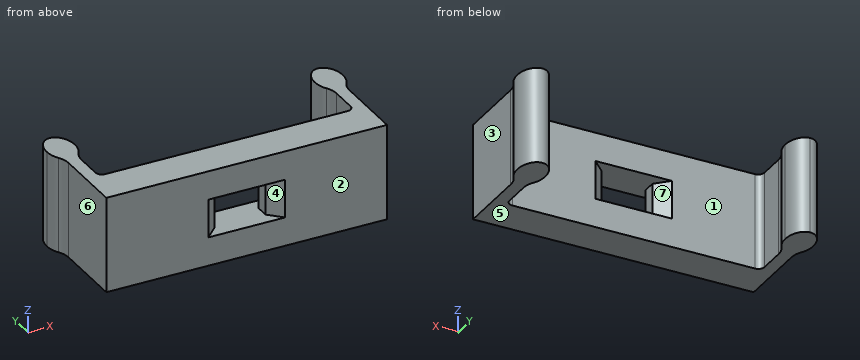
Autodesk Fusion 360 part; units mm, degrees
sketch "Sketch1" plane through (0, 0, 0) normal (0, 0, 1) x (1, 0, 0) in component "Ender5RailClip"
  line L0 (-21.0864, 9.1534) -> (22.9136, 9.1534)
  line L1 (22.9136, 9.1534) -> (22.9136, 3.1534)
  line L2 (22.9136, 3.1534) -> (-21.0864, 3.1534)
  line L3 (-21.0864, 3.1534) -> (-21.0864, 9.1534)
  line L4 (-21.0864, 9.1534) -> (-19.0864, 9.1534)
  line L5 (-19.0864, 9.1534) -> (-19.0864, 16)
  line L6 (-19.0864, 16) -> (-21.0864, 16)
  line L7 (-21.0864, 16) -> (-21.0864, 9.1534)
  line L8 (0.9136, 9.1534) -> (0.9136, 18) construction
  ellipse E0 centre (-20.0864, 18.5) end of major axis (-20.0864, 15.25) minor radius 2.2
  line L9 (-20.0864, 21.75) -> (-20.0864, 15.25)
  line L10 (-22.2864, 18.5) -> (-17.8864, 18.5)
  ellipse E1 centre (21.9136, 18.5) end of major axis (21.9136, 15.25) minor radius 2.2
  line L11 (20.9136, 16) -> (22.9136, 16)
  line L12 (20.9136, 9.1534) -> (20.9136, 16)
  line L13 (22.9136, 16) -> (22.9136, 9.1534)
  point P0 (-20.0864, 16)
  dimension "d2" = 6
  dimension "d3" = 2
  dimension "d4" = 6.5
  dimension "d5" = 4.4
  dimension "d6" = 2.5
  dimension "d19" = 40
extrude "Extrude1" add sketch "Sketch1" along normal blind 15 in component "Ender5RailClip"
fillet "Fillet1" radius 1 2 edges at (20.9136, 9.1534, 7.5) (-19.0864, 9.1534, 7.5) in component "Ender5RailClip"
fillet "Fillet2" radius 3.5 4 edges at (-19.0864, 15.6051, 7.5) (20.9136, 15.6051, 7.5) (-21.0864, 15.6051, 7.5) (22.9136, 15.6051, 7.5) in component "Ender5RailClip"
sketch "Sketch2" plane through (0, 3.1534, 0) normal (0, -1, 0) x (1, 0, 0) in component "Ender5RailClip"
  line L0 (-21.0864, 0) -> (22.9136, 0)
  line L1 (22.9136, 0) -> (22.9136, 15)
  line L2 (22.9136, 15) -> (-21.0864, 15)
  line L3 (-21.0864, 15) -> (-21.0864, 0)
  line L4 (0.9136, 0) -> (0.9136, 15) construction
  line L5 (-21.0864, 7.5) -> (22.9136, 7.5) construction
  line L6 (4.9136, 4.5) -> (-3.0864, 4.5)
  line L7 (-3.0864, 4.5) -> (-3.0864, 10.5)
  line L8 (-3.0864, 10.5) -> (4.9136, 10.5)
  line L9 (4.9136, 10.5) -> (4.9136, 4.5)
  line L10 (4.9136, 4.5) -> (-3.0864, 10.5) construction
  line L11 (-3.0864, 4.5) -> (4.9136, 10.5) construction
  point P0 (0.9136, 7.5)
  dimension "d20" = 8
  dimension "d21" = 6
extrude "Extrude3" cut sketch "Sketch2" against normal through all contours L6 L7 L8 L9 in component "Ender5RailClip"
chamfer "Chamfer2" distance 2 angle 45 4 edges at (-3.0864, 9.1534, 7.5) (-3.0864, 3.1534, 7.5) (4.9136, 9.1534, 7.5) (4.9136, 3.1534, 7.5) in component "Ender5RailClip"
component "Ender5RailClip" placed x (1, 0, 0) y (0, 1, 0) z (0, 0, 1) at (0, 0, 0)
CAD build for the part. Positions are in the model's coordinates, mm. Face numbers are marked on the shaded views. A direction names the side the tool comes from. Round coordinates to 2 decimals unless told otherwise and drop trailing zeros. Write each loop counter-clockwise with the first axis right and the second up, starting at its lowest first coordinate (ties: lowest second). Pieces come first, ordered by that corner, then holes.
(1) Probe line 1 along Z through (x, y) = (0.5, 6.5); line 2 along X through (y, z) = (11.75, 8.5); line 3 along Y through (x, z) = (-7.5, 2.75). List the from-to ranges inside material, lowest first.
(2) Slice it at A-A, the plane y = 11. Write the cut outline in (x, z).
(3) Drop flat-ended pins along their axis: P1, Ø6, axis at x = -7, y = 15, coming from the -Z side; P2, Ø2, axis at y = 10.5, z = 9, coming from the -X side; P3, Ø1.5, axis at y = 20, z = 6, coming from the -X side; P4, Ø4.5, axis at x = 6, z = 6.5, coming from the +Y side. Give the stop position or say it passes through.
(4) Slice it at B-B, the plane y = 5.75. Write the cut outline in (x, z), and give its area (3 significant figures).
(5) Mould opens along X. For the marked faces 1, 2, 3 and 4 say: pulls with the +X half, pulls with the -X half, needs draft (parallel to the pull), parting line crosses it, or undercut.
(6) 3-axis set-ups, long thin cutter, end or side, ignore diameter. For the marked faces 5, 6 and 7: which of +Z, -Z, +X, -X, +Y, -Y reach the whole face in a straight line?
(7) Slice it at D-D, the plane y = 8.5. Write the cut outline in (x, z), and give its area (3 significant figures).
(8) Slice it at C-C, the plane x = -4. Write the cut outline in (y, z), and give its area (3 significant figures).
From the geometry:
1. line 1: z = 0 to 4.5, 10.5 to 15
1. line 2: x = -21.09 to -19.09, 20.91 to 22.91
1. line 3: y = 3.15 to 9.15
2. outline: (-21.09, 0) - (-19.09, 0) - (-19.09, 15) - (-21.09, 15) - close; (20.91, 0) - (22.91, 0) - (22.91, 15) - (20.91, 15) - close
3. P1: passes through
3. P2: stops at x = -21.09
3. P3: stops at x = -22.23
3. P4: stops at y = 9.15
4. outline: (-21.09, 0) - (22.91, 0) - (22.91, 15) - (-21.09, 15) - close; hole (-3.09, 4.5) - (4.91, 4.5) - (4.91, 10.5) - (-3.09, 10.5) - close
4. area: 612 mm2
5. face 1: undercut
5. face 2: needs draft
5. face 3: pulls with the +X half
5. face 4: undercut
6. face 5: -Z, +X, -X, +Y, -Y
6. face 6: +Z, -Z, -X, -Y
6. face 7: +Y
7. outline: (-21.09, 0) - (22.91, 0) - (22.91, 15) - (-21.09, 15) - close; hole (-4.43, 4.5) - (6.26, 4.5) - (6.26, 10.5) - (-4.43, 10.5) - close
7. area: 596 mm2
8. outline: (3.15, 0) - (9.15, 0) - (9.15, 4.5) - (8.07, 4.5) - (8.07, 10.5) - (9.15, 10.5) - (9.15, 15) - (3.15, 15) - (3.15, 10.5) - (4.24, 10.5) - (4.24, 4.5) - (3.15, 4.5) - close
8. area: 77.0 mm2
